```python
from build123d import *

# Parameters (mm, degrees)
SKETCH1_W           = 70
SKETCH1_H           = 105
BOSS_EXTRUDE1_DEPTH = 2
SKETCH2_R           = 17.5
CUT_EXTRUDE3_DEPTH  = 3
CUT_EXTRUDE6_DEPTH  = 10
SCALE1_SCALE        = 1.771428571
SKETCH6_R           = 30.999999993
CUT_EXTRUDE7_DEPTH  = 0.31
SKETCH7_W           = 123.99999997
SKETCH7_H           = 38.57142855
CUT_EXTRUDE8_DEPTH  = 10
SKETCH9_R           = 2.5
CUT_EXTRUDE9_DEPTH  = 3.232857142
SKETCH10_R          = 2.5
CUT_EXTRUDE10_DEPTH = 3.232857142


with BuildPart() as part:
    # Sketch1 → Boss-Extrude1 (new body)
    with BuildSketch(Plane.XY):
        Rectangle(SKETCH1_W, SKETCH1_H)
    extrude(amount=BOSS_EXTRUDE1_DEPTH)

    # Sketch2 → Cut-Extrude3 (cut)
    with BuildSketch(Plane(origin=(0, 0, 0), x_dir=(-1, 0, 0), z_dir=(0, 0, -1))):
        with Locations((0, 20.5)):
            Circle(SKETCH2_R)
    extrude(amount=-CUT_EXTRUDE3_DEPTH, mode=Mode.SUBTRACT)

    # Sketch5 → Cut-Extrude6 (cut)
    with BuildSketch(Plane.XY.offset(2)):
        with BuildLine():
            Line((-35, 40.793543502), (-35, 52.5))
            Line((-35, 52.5), (35, 52.5))
            Line((35, 52.5), (35, 40.793543502))
            ThreePointArc((35, 40.793543502), (0, 48.07644174), (-35, 40.793543502))
        make_face()
    extrude(amount=-CUT_EXTRUDE6_DEPTH, mode=Mode.SUBTRACT)


with BuildPart() as part_1:
    # Scale1: scaled about (0, -7.267874882, 1)
    add(part.part.scale(SCALE1_SCALE).moved(Location((0, 5.606646334, -0.771428571))))

    # Sketch6 → Cut-Extrude7 (cut)
    with BuildSketch(Plane(origin=(0, 0, -0.771428571), x_dir=(-1, 0, 0), z_dir=(0, 0, -1))):
        with BuildLine():
            Line((61.999999985, -87.393353643), (61.999999985, 77.869494806))
            ThreePointArc((61.999999985, 77.869494806), (0, 90.770628825), (-61.999999985, 77.869494806))
            Line((-61.999999985, 77.869494806), (-61.999999985, -87.393353643))
            Line((-61.999999985, -87.393353643), (61.999999985, -87.393353643))
        make_face()
        with Locations((0, 41.92093204)):
            Circle(SKETCH6_R, mode=Mode.SUBTRACT)
    extrude(amount=-CUT_EXTRUDE7_DEPTH, mode=Mode.SUBTRACT)

    # Sketch7 → Cut-Extrude8 (cut)
    with BuildSketch(Plane.XY.offset(2.771428571)):
        with Locations((0, -68.107639368)):
            Rectangle(SKETCH7_W, SKETCH7_H)
    extrude(amount=-CUT_EXTRUDE8_DEPTH, mode=Mode.SUBTRACT)

    # Sketch9 → Cut-Extrude9 (cut)
    with BuildSketch(Plane.XY.offset(2.771428571)):
        with Locations((0, -38.821925093)):
            Circle(SKETCH9_R)
        with Locations((-23, -13.821925093)):
            Circle(SKETCH9_R)
        with Locations(Location((23, -13.821925093, 0), (0, 0, 180))):
            Circle(SKETCH9_R)
    extrude(amount=-CUT_EXTRUDE9_DEPTH, mode=Mode.SUBTRACT)

    # Sketch10 → Cut-Extrude10 (cut)
    with BuildSketch(Plane.XY.offset(2.771428571)):
        with Locations((-40.233402491, 44.236817184)):
            Circle(SKETCH10_R)
        with Locations((0, 82.22093204)):
            Circle(SKETCH10_R)
        with Locations((40.233400771, 44.236847056)):
            Circle(SKETCH10_R)
    extrude(amount=-CUT_EXTRUDE10_DEPTH, mode=Mode.SUBTRACT)


solid = part_1.part
```
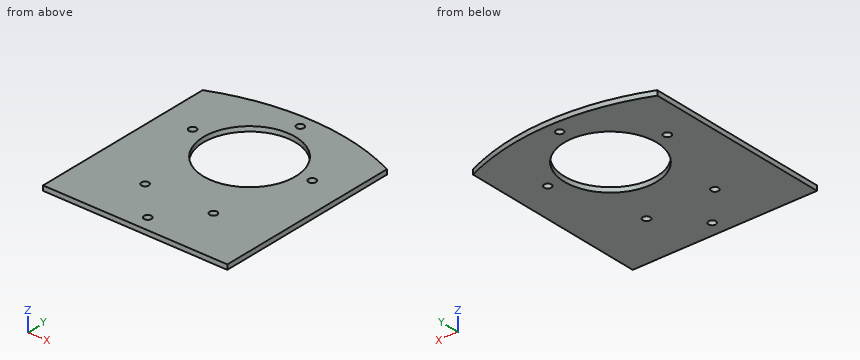
CAD build for the part. Positions are in the model's coordinates, mm. Round coordinates to 2 decimals unless told otherwise and drop trailing zeros. Loops run counter-clockwise (first coordinate to the right, second up) from the corner with the lowest first, then second, coordinate; pieces in that order, holes last. Notation, with made-up numbers: M -38.75,-30.75 L -3.75,-30.75 A17 cw -3.75,-12.75 Z; hole C 14,83 d2. An arc over 180 degrees is marked long. Return JSON: item names as keys, results as strings. Group by question number.
(1) Saw through at B-B, the plane y = 39. List the corners of the cut face in (x, z).
(2) Saw through at A-A, the plane x = 0. List the corners of the cut face in (y, z), and give its area (3 significant figures).
(3) Drop flat-ended pins along their axis: P1, Ø8, axis at x = 23, y = -13.82, coming from the -Z side; P2, Ø4.5, axis at x = 0, y = 82.22, coming from the -Z side. Give the stop position or say it passes through.
(4) Saw through at C-C, the plane z = 0.3. List the corners of the cut face in (x, y).
(5) Saw through at D-D, the plane x = 24. List the corners of the cut face in (y, z).
(6) Wall check: probe 1 along X at (y, z) = (-14, 1.65); probe 2 along Y at (x, z) = (0, 1.75); probe 3 along Y at (x, z) = (-23, 1). Give the ranges that are in metal, low to high. Write a range as [from, to].
Answer list:
{
 "1": {"outline": "M -62,-0.46 L -30.86,-0.46 L -30.86,2.77 L -62,2.77 Z; M 30.86,-0.46 L 62,-0.46 L 62,2.77 L 30.86,2.77 Z"},
 "2": {"outline": "M -48.82,-0.46 L -41.32,-0.46 L -41.32,2.77 L -48.82,2.77 Z; M -36.32,-0.46 L 10.92,-0.46 L 10.92,2.77 L -36.32,2.77 Z; M 72.92,-0.46 L 79.72,-0.46 L 79.72,2.77 L 72.92,2.77 Z; M 84.72,-0.46 L 90.77,-0.46 L 90.77,2.77 L 84.72,2.77 Z", "area": "219 mm2"},
 "3": {"P1": "z = -0.46", "P2": "through"},
 "4": {"outline": "M -62,-48.82 L 62,-48.82 L 62,77.87 A155.43 ccw -62,77.87 Z; hole C -40.23,44.24 d5; hole C 0,41.92 d62; hole C -23,-13.82 d5; hole C 0,-38.82 d5; hole C 0,82.22 d5; hole C 23,-13.82 d5; hole C 40.23,44.24 d5"},
 "5": {"outline": "M -48.82,-0.46 L -16.11,-0.46 L -16.11,2.77 L -48.82,2.77 Z; M -11.53,-0.46 L 22.3,-0.46 L 22.3,2.77 L -11.53,2.77 Z; M 61.54,-0.46 L 88.91,-0.46 L 88.91,2.77 L 61.54,2.77 Z"},
 "6": {"probe 1": "[-62, -25.49], [-20.51, 20.51], [25.49, 62]", "probe 2": "[-48.82, -41.32], [-36.32, 10.92], [72.92, 79.72], [84.72, 90.77]", "probe 3": "[-48.82, -16.32], [-11.32, 21.14], [62.71, 89.06]"}
}
